Model file for the job. Use its own axes, mm. A direction names the side the tool comes from. Coordinates: 2 decimals unless noted, no trailing zeros. Write each loop counter-clockwise with the first axis right and the second up, starting at its lowest first coordinate (ties: lowest second). Pieces come first, ordered by that corner, then holes. Notation, with made-up numbers: (11.25, 36) -> (26.25, 36) arc R21 ccw to (26.25, 40) -> close; hole circle Ø9 at (66.5, 88). An arc over 180 degrees is marked (long way). Write item = value, one per line. Start each with the question number.
from build123d import *

# Parameters (mm, degrees)
SKETCH1_W           = 20
SKETCH1_H           = 20
BOSS_EXTRUDE1_DEPTH = 8.5
CUT_EXTRUDE1_DEPTH  = 34
SKETCH3_W           = 13
SKETCH3_H           = 17
CUT_EXTRUDE2_DEPTH  = 17
CUT_EXTRUDE4_DEPTH  = 28.590759323
CUT_EXTRUDE5_DEPTH  = 28.590759323
SKETCH7_W           = 4.5
SKETCH7_H           = 1.6
BOSS_EXTRUDE2_DEPTH = 1
SKETCH8_W           = 4.5
SKETCH8_H           = 1.6
BOSS_EXTRUDE3_DEPTH = 1


with BuildPart() as part:
    # Sketch1 → Boss-Extrude1 (new, symmetric)
    with BuildSketch(Plane(origin=(0, 0, 0), x_dir=(0, 0, -1), z_dir=(1, 0, 0))):
        with Locations((-10, 10)):
            Rectangle(SKETCH1_W, SKETCH1_H)
    extrude(amount=BOSS_EXTRUDE1_DEPTH, both=True)

    # Sketch2 → Cut-Extrude1 (cut, through all)
    with BuildSketch(Plane.ZY.offset(8.5)):
        Polygon((20, 20), (3, 20), (20, 3), align=None)
    extrude(amount=-CUT_EXTRUDE1_DEPTH, mode=Mode.SUBTRACT)

    # Sketch3 → Cut-Extrude2 (cut)
    with BuildSketch(Plane(origin=(0, 20, 0), x_dir=(1, 0, 0), z_dir=(0, 1, 0))):
        with Locations((0, -11.5)):
            Rectangle(SKETCH3_W, SKETCH3_H)
    extrude(amount=-CUT_EXTRUDE2_DEPTH, mode=Mode.SUBTRACT)

    # Sketch5 → Cut-Extrude4 (cut, through all)
    with BuildSketch(Plane.XY.offset(3)):
        with BuildLine():
            Line((-3.3, 9), (-3.3, 12))
            ThreePointArc((-3.3, 12), (0, 15.3), (3.3, 12))
            Line((3.3, 12), (3.3, 9))
            ThreePointArc((3.3, 9), (0, 5.7), (-3.3, 9))
        make_face()
    extrude(amount=-CUT_EXTRUDE4_DEPTH, mode=Mode.SUBTRACT)

    # Sketch6 → Cut-Extrude5 (cut, through all)
    with BuildSketch(Plane(origin=(0, 3, 0), x_dir=(1, 0, 0), z_dir=(0, 1, 0))):
        with BuildLine():
            Line((3.3, -9), (3.3, -12))
            ThreePointArc((3.3, -12), (0, -15.3), (-3.3, -12))
            Line((-3.3, -12), (-3.3, -9))
            ThreePointArc((-3.3, -9), (0, -5.7), (3.3, -9))
        make_face()
    extrude(amount=-CUT_EXTRUDE5_DEPTH, mode=Mode.SUBTRACT)

    # Sketch7 → Boss-Extrude2 (add)
    with BuildSketch(Plane(origin=(0, 0, 0), x_dir=(-1, 0, 0), z_dir=(0, 0, -1))):
        with Locations((0, 17.8)):
            Rectangle(SKETCH7_W, SKETCH7_H)
        with Locations((0, 2.2)):
            Rectangle(SKETCH7_W, SKETCH7_H)
    extrude(amount=BOSS_EXTRUDE2_DEPTH)

    # Sketch8 → Boss-Extrude3 (add)
    with BuildSketch(Plane.XZ):
        with Locations((0, 17.8)):
            Rectangle(SKETCH8_W, SKETCH8_H)
        with Locations((0, 2.2)):
            Rectangle(SKETCH8_W, SKETCH8_H)
    extrude(amount=BOSS_EXTRUDE3_DEPTH)


solid = part.part
(1) 3-axis set-ups, long thin cutter, end or side, ignore diameter. For faces 4 (the face through (-2.25, -0.5, 2.2)), 5 (the face through (0.1, 5.7, 1.5)), 6 (the face through (0, 3, -0.5)): which of +Z, -Z, +X, -X, +Y, -Y reach the whole face in a straight line?
(2) Mould opens along X. For faces 1 (the face through (2.25, 2.2, -0.5)), 2 (the face through (0.1, 1.5, 15.3)), 3 (the face through (-2.25, 17.8, -0.5)) say: released by +X, released by -X, zero draft, split by the parting line, or undercut.
(3) Drop flat-ended pins along their axis: pin 1 Ø1 at (x, y) = (-1.5, 7.5) entering from -Z; pin 2 Ø0.5 at (y, z) = (18, -0.5) entering from +X; pin 3 Ø1.1 at (y, z) = (2, -0.5) entering from +X; pin 4 Ø8 at (x, y) = (-4.5, 10.5) entering from -Z. Give the stop position or say it passes through.
(4) Saw through at A-A (z = 9.5). Give the cut face in (x, y), then the cut area to 3 significant figures.
(5) Saw through at D-D (z = 4). Give the cut face in (x, y).
(6) Drill centre lines: line 1 along X through (y, z) = (12.25, 8); line 2 along X through (y, z) = (11.5, 2.5); line 3 along Y through (x, z) = (2.5, 6.25). Where is each one in solid material? Low to high.
(7) Saw through at C-C (x = 0). State how many separate pieces and enclosed holes the cut face has, then the cut area to 3 significant figures.
Returned:
q1.face_4 = +Z, -Z, -X, -Y
q1.face_5 = +Z, -Z
q1.face_6 = -Z, +X, -X
q2.face_1 = released by +X
q2.face_2 = undercut
q2.face_3 = released by -X
q3.pin_1 = through
q3.pin_2 = 2.25
q3.pin_3 = 8.5
q3.pin_4 = 0
q4.outline = (-8.5, 0) -> (-3.3, 0) -> (-3.3, 3) -> (-6.5, 3) -> (-6.5, 13.5) -> (-8.5, 13.5) -> close; (3.3, 0) -> (8.5, 0) -> (8.5, 13.5) -> (6.5, 13.5) -> (6.5, 3) -> (3.3, 3) -> close
q4.area = 73.2 mm2
q5.outline = (-8.5, 0) -> (8.5, 0) -> (8.5, 19) -> (6.5, 19) -> (6.5, 3) -> (-6.5, 3) -> (-6.5, 19) -> (-8.5, 19) -> close
q6.line_1 = -8.5 to -6.5, 6.5 to 8.5
q6.line_2 = -8.5 to -3.3, 3.3 to 8.5
q6.line_3 = 0 to 3
q7.separate_pieces = 3
q7.enclosed_holes = 0
q7.area = 59.8 mm2
